```python
from build123d import *


with BuildPart() as part:
    # Sweep1: sweep along a path in Sketch1
    with BuildLine(Plane(origin=(0, 0, 0), x_dir=(1, 0, 0), z_dir=(0, 1, 0))) as sweep1_path:
        Line((0, 0), (-51.975, 0))
        ThreePointArc((-51.975, 0), (-53.389213562, -0.585786438), (-53.975, -2))
        Line((-53.975, -2), (-53.975, -19.05))
    # Sketch2 → Sweep1 (sweep)
    with BuildSketch(Plane(origin=(0, 0, 0), x_dir=(0, 0, -1), z_dir=(1, 0, 0))):
        Polygon((1.25, -0.721687836), (2.5, 0), (2.5, 1.443375673), (1.25, 2.165063509), (0, 1.443375673), (0, 0), align=None)
    sweep(path=sweep1_path.line)


solid = part.part
```
Input: part model. Units: mm. Frame: model coordinates. A direction names the side the tool comes from. Round coordinates to 2 decimals unless told otherwise and drop trailing zeros. Loops run counter-clockwise (first coordinate to the right, second up) from the corner with the lowest first, then second, coordinate; pieces in that order, holes last. Notation, with made-up numbers: M 23.5,-13 L 60.5,-13 A21 cw 60.5,-3 Z; hole C -38,-17 d8. An arc over 180 degrees is marked long. Answer in a Markdown table with one row per item. Add a question column.
1. Section A-A (z = 10.5). Output: boundary loops of the cut face in (x, y) (3 decimals), and give its area (3 significant figures).
2. Set-up query: faces 1 (the face through (0, 1, -1)), 2 (the face through (-26.351, 1.809, -0.634)), 3 (the face through (-26, 1, 0)), 4 (the face through (-26, 1, -2.5)), 5 (the face through (-54.591, -0.356, 10.644)). Return all of +Z, -Z, +X, -X, +Y, -Y with unobstructed straight access to the full face (end or side cutting, diameter ignored); none if empty.
3. Ray query, probe 1 along X at (y, z) = (1.3, 12.25) (3 decimals); probe 2 along Z at (x, y) = (-39.5, 1.25); probe 3 along X at (y, z) = (1.7, 17.75). Return the intervals inside material, ascending.
4. Contact query for flat-ended pins moving along their axis: pin 1 (6 mm diameter, centred on x = -49.5, z = 0, fed in from -Y); pin 2 (1.2 mm diameter, centred on x = -28, y = 1, fed in from +Z). Output: stop coordinate, or through.
5. Section B-B (y = 0.7). Output: boundary loops of the cut face in (x, z) (3 decimals), and give its area (3 significant figures).
6. Section C-C (x = -22). Output: boundary loops of the cut face in (y, z).
Values follow:
| question | item | result |
|---|---|---|
| 1 | outline | M -56.475,0 L -55.225,-0.722 L -53.975,0 L -53.975,1.443 L -55.225,2.165 L -56.475,1.443 Z |
| 1 | area | 5.41 mm^2 |
| 2 | face 1 | +Z, -Z, +X, +Y, -Y |
| 2 | face 2 | +Z, +X, +Y |
| 2 | face 3 | +Z, +X, +Y, -Y |
| 2 | face 4 | -Z, +X, -X, +Y, -Y |
| 2 | face 5 | +Z, +X, -Y |
| 3 | probe 1 | -56.475 to -53.975 |
| 3 | probe 2 | -2.5 to 0 |
| 3 | probe 3 | -56.03 to -54.42 |
| 4 | pin 1 | y = -0.72 |
| 4 | pin 2 | z = 0 |
| 5 | outline | M -56.475,2 A4.5 ccw -51.975,-2.5 L 0,-2.5 L 0,0 L -51.975,0 A2 cw -53.975,2 L -53.975,19.05 L -56.475,19.05 Z |
| 5 | area | 185 mm^2 |
| 6 | outline | M -0.72,-1.25 L 0,-2.5 L 1.44,-2.5 L 2.17,-1.25 L 1.44,0 L 0,0 Z |
